from build123d import *

# Parameters (mm, degrees)
SKETCH1_W           = 155
SKETCH1_H           = 65
BOSS_EXTRUDE1_DEPTH = 1.5
SKETCH2_W           = 145
SKETCH2_H           = 55
SKETCH2_W_2         = 139
SKETCH2_H_2         = 49
BOSS_EXTRUDE2_DEPTH = 10
CUT_EXTRUDE1_DEPTH  = 91
SKETCH5_R           = 3
SKETCH5_R_2         = 4
SKETCH5_W           = 45.5
SKETCH5_H           = 27
CUT_EXTRUDE2_DEPTH  = 91
SKETCH6_R           = 1.5
CUT_EXTRUDE3_DEPTH  = 91


with BuildPart() as part:
    # Sketch1 → Boss-Extrude1 (new body)
    with BuildSketch(Plane(origin=(0, 0, 0), x_dir=(1, 0, 0), z_dir=(0, 1, 0))):
        with Locations((-3.071428571, 5.285714286)):
            Rectangle(SKETCH1_W, SKETCH1_H)
    extrude(amount=BOSS_EXTRUDE1_DEPTH)

    # Sketch2 → Boss-Extrude2 (add)
    with BuildSketch(Plane(origin=(0, 1.5, 0), x_dir=(1, 0, 0), z_dir=(0, 1, 0))):
        with Locations((-3.071428571, 5.285714286)):
            Rectangle(SKETCH2_W, SKETCH2_H)
        with Locations((-3.071428571, 5.285714286)):
            Rectangle(SKETCH2_W_2, SKETCH2_H_2, mode=Mode.SUBTRACT)
    extrude(amount=BOSS_EXTRUDE2_DEPTH)

    # Sketch4 → Cut-Extrude1 (cut)
    with BuildSketch(Plane.XY.offset(22.214285714)):
        Polygon((-65.571428571, 11.5), (-63.571428571, 6.5), (-23.571428571, 6.5), (-18.571428571, 11.5), align=None)
        Polygon((4.928571429, 11.5), (59.428571429, 11.5), (46.928571429, 6.5), (6.928571429, 6.5), align=None)
    extrude(amount=-CUT_EXTRUDE1_DEPTH, mode=Mode.SUBTRACT)

    # Sketch5 → Cut-Extrude2 (cut)
    with BuildSketch(Plane.XZ):
        with Locations(Location((16.687112177, -24.986454546, 0), (0, 0, 270))):
            Circle(SKETCH5_R)
        with Locations(Location((31.687110951, -24.980390104, 0), (0, 0, 270))):
            Circle(SKETCH5_R)
        with Locations(Location((55.455936184, -0.234986803, 0), (0, 0, 270))):
            Circle(SKETCH5_R_2)
        with Locations(Location((-12.375354301, 0.783116326, 0), (0, 0, 270))):
            Circle(SKETCH5_R_2)
        with Locations(Location((-56.616849976, -24.986454546, 0), (0, 0, 270))):
            Circle(SKETCH5_R)
        with Locations(Location((-41.616849976, -24.986454546, 0), (0, 0, 270))):
            Circle(SKETCH5_R)
        with Locations((20.705936184, -1.486454546)):
            Rectangle(SKETCH5_W, SKETCH5_H)
        with Locations((-47.125354301, -1.486454546)):
            Rectangle(SKETCH5_W, SKETCH5_H)
    extrude(amount=-CUT_EXTRUDE2_DEPTH, mode=Mode.SUBTRACT)

    # Sketch6 → Cut-Extrude3 (cut)
    with BuildSketch(Plane.XY.offset(22.214285714)):
        with Locations((-8.074390062, 8.312033368)):
            Circle(SKETCH6_R)
        with Locations((61.496987575, 8.312033368)):
            Circle(SKETCH6_R)
        with Locations((-68.65, 8.3)):
            Circle(SKETCH6_R)
    extrude(amount=-CUT_EXTRUDE3_DEPTH, mode=Mode.SUBTRACT)


solid = part.part
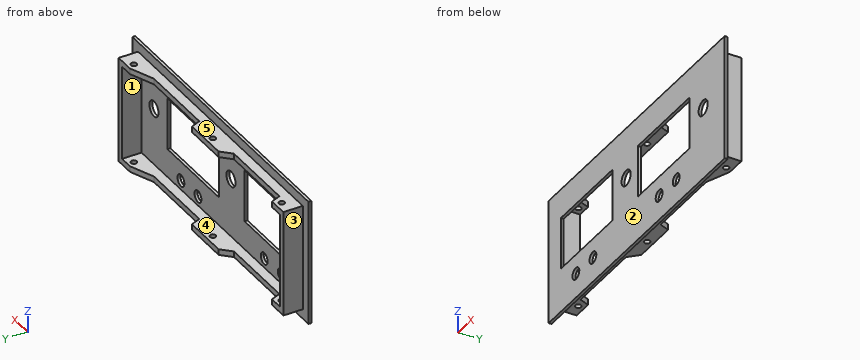
Source: CAD feature listing. Evaluate the final solid. Frame: model axes, mm. Face numbers are marked on the shaded views. A direction names the side the tool comes from. Coordinates: 2 decimals unless noted, no trailing zeros. Write each loop counter-clockwise with the first axis right and the second up, starting at its lowest first coordinate (ties: lowest second). Pieces come first, ordered by that corner, then holes. Notation, with made-up numbers: M 51.25,13 L 66.25,13 A13 ccw 66.25,23 Z; hole C 78,66.25 d3. An arc over 180 degrees is marked long. Use a Markdown table: item, result.
1) Section B-B, the plane x = -50.5. Output: boundary loops of the cut face in (y, z).
Conclusion:
| item | result |
|---|---|
| outline | M 0,-37.79 L 1.5,-37.79 L 1.5,-32.79 L 6.5,-32.79 L 6.5,-29.79 L 1.5,-29.79 L 1.5,-14.99 L 0,-14.99 Z; M 0,12.01 L 1.5,12.01 L 1.5,19.21 L 6.5,19.21 L 6.5,22.21 L 1.5,22.21 L 1.5,27.21 L 0,27.21 Z |
2) Section C-C, the plane z = -20.5. Output: boundary loops of the cut face in (x, y).
Conclusion:
| item | result |
|---|---|
| outline | M -80.57,0 L 74.43,0 L 74.43,1.5 L 69.43,1.5 L 69.43,11.5 L 66.43,11.5 L 66.43,1.5 L -72.57,1.5 L -72.57,11.5 L -75.57,11.5 L -75.57,1.5 L -80.57,1.5 Z |
3) Reachability of the marked faces 1 and 2 from +Z, -Z, +X, -X, +Y, -Y: full face, straight path, thin tool, end or side. Return the list, or none.
Conclusion:
| item | result |
|---|---|
| face 1 | +Y |
| face 2 | +Z, -Z, +X, -X, -Y |
4) Section A-A, the plane y = 3.25. Output: boundary loops of the cut face in (x, z).
Conclusion:
| item | result |
|---|---|
| outline | M -75.57,-32.79 L 69.43,-32.79 L 69.43,22.21 L -75.57,22.21 Z; hole M -72.57,-29.79 L 66.43,-29.79 L 66.43,19.21 L -72.57,19.21 Z |
5) Ray query, L1, parallel to X at y = 6, z = -2.5; L2, parallel to Z at x = -14, y = 11; L3, parallel to Y at x = 2.5, z = -24.5. Return the intervals inside material, ascending.
Conclusion:
| item | result |
|---|---|
| L1 | x = -75.57 to -72.57, 66.43 to 69.43 |
| L2 | z = -32.79 to -29.79, 19.21 to 22.21 |
| L3 | y = 0 to 1.5 |
6) First-contact query: pin 1 Ø3 at (x, y) = (-13, 6.5) entering from -Z; pin 2 Ø3.5 at (x, z) = (-46, -32) entering from +Y; pin 3 Ø4 at (x, y) = (61.5, 8.31) entering from +Z; pin 4 Ø3 at (x, y) = (-30.5, 9.5) entering from -Z. Flat tips, straight axial feed; report the tip coordinate or a pass-through.
Conclusion:
| item | result |
|---|---|
| pin 1 | stops at z = -32.79 |
| pin 2 | stops at y = 6.5 |
| pin 3 | stops at z = 22.21 |
| pin 4 | passes through |
7) Section D-D, the plane x = 65. Output: boundary loops of the cut face in (y, z).
Conclusion:
| item | result |
|---|---|
| outline | M 0,-37.79 L 1.5,-37.79 L 1.5,-32.79 L 11.5,-32.79 L 11.5,-29.79 L 1.5,-29.79 L 1.5,19.21 L 11.5,19.21 L 11.5,22.21 L 1.5,22.21 L 1.5,27.21 L 0,27.21 Z |
8) Mould query, pull axis Z, two halves, no side actions, for the marked faces 3, 4 and 5. Classes: pulls with the +Z half, pulls with the -Z half, needs draft (parallel to the pull), parting line crosses it, or undercut.
Conclusion:
| item | result |
|---|---|
| face 3 | needs draft |
| face 4 | undercut |
| face 5 | pulls with the +Z half |
